from build123d import *

# Parameters (mm, degrees)
BOARD_START    = 10
BOARD_DEPTH    = 1.6
TERMINAL_START = 11.6
SKETCH2_W      = 10
SKETCH2_H      = 7.5
TERMINAL_DEPTH = 10


with BuildPart() as part:
    # Sketch1 → Board (new body)
    with BuildSketch(Plane(origin=(0, 0, 0), x_dir=(1, 0, 0), z_dir=(0, 1, 0)).offset(BOARD_START)):
        with BuildLine():
            Line((-56, -21), (-38, -21))
            ThreePointArc((-38, -21), (-37.292893219, -21.292893219), (-37, -22))
            Line((-37, -22), (-37, -38))
            ThreePointArc((-37, -38), (-37.292893219, -38.707106781), (-38, -39))
            Line((-38, -39), (-56, -39))
            ThreePointArc((-56, -39), (-56.707106781, -38.707106781), (-57, -38))
            Line((-57, -38), (-57, -22))
            ThreePointArc((-57, -22), (-56.707106781, -21.292893219), (-56, -21))
        make_face()
    extrude(amount=BOARD_DEPTH)

    # Sketch2 → Terminal (add)
    with BuildSketch(Plane(origin=(0, 0, 0), x_dir=(1, 0, 0), z_dir=(0, 1, 0)).offset(TERMINAL_START)):
        with Locations((-47, -34)):
            Rectangle(SKETCH2_W, SKETCH2_H)
    extrude(amount=TERMINAL_DEPTH)


solid = part.part
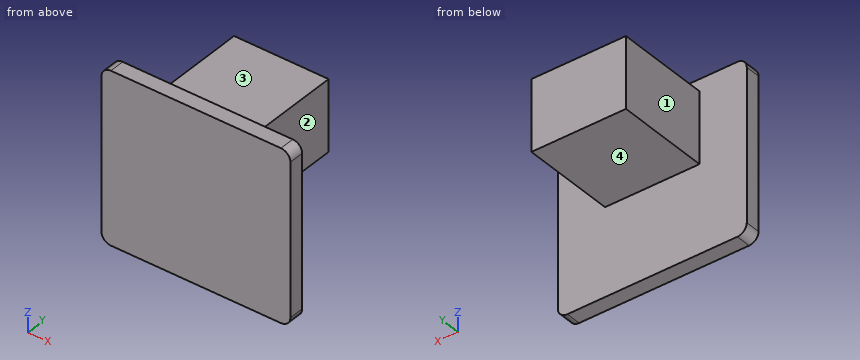
Geometry: final body of the model. Coordinates: model frame, mm. Face numbers are marked on the shaded views. A direction names the side the tool comes from. Round coordinates to 2 decimals unless told otherwise and drop trailing zeros. Order: outer loops, then holes, each group sorted by start corner. A loop starts at its lowest first (then second) coordinate and runs counter-clockwise, first axis right, second up. Notation, with made-up numbers: (2.25, 57) -> (55.25, 57) arc R11 cw to (55.25, 75) -> close; hole circle Ø8 at (88.5, 37.5). An arc over 180 degrees is marked (long way). Put each result on its own line as item: value. Start each with the question number.
Q1. Section B-B on x = -51.75. Return the cut outline in (y, z).
Q2. Section A-A on z = 33.25. Return the cut outline in (x, y), and give its area (3 significant figures).
Q3. Section C-C on y = 16.75. Return the cut outline in (x, z).
Q4. Reachability of the marked faces 1, 2, 3 and 4 from +Z, -Z, +X, -X, +Y, -Y: full face, straight path, thin tool, end or side. Return the list, or none.
Q5. Section D-D on z = 28.5. Return the cut outline in (x, y).
Q6. Line query: probe 1 along Z at (x, y) = (-48.25, 15.75); probe 2 along Y at (x, z) = (-49, 29); probe 3 along X at (y, z) = (12.25, 32). Output: solid intervals per line, ascending.
Q7. First-contact query: pin 1 (2 mm diameter, centred on y = 18, z = 32.5, fed in from +X); pin 2 (3 mm diameter, centred on x = -49, y = 17, fed in from +Z). Flat tips, straight axial feed; report the tip coordinate or a pass-through.
Ans:
1. outline: (10, 21) -> (11.6, 21) -> (11.6, 30.25) -> (21.6, 30.25) -> (21.6, 37.75) -> (11.6, 37.75) -> (11.6, 39) -> (10, 39) -> close
2. outline: (-57, 10) -> (-37, 10) -> (-37, 11.6) -> (-42, 11.6) -> (-42, 21.6) -> (-52, 21.6) -> (-52, 11.6) -> (-57, 11.6) -> close
2. area: 132 mm2
3. outline: (-52, 30.25) -> (-42, 30.25) -> (-42, 37.75) -> (-52, 37.75) -> close
4. face 1: +Z, -Z, -X, +Y
4. face 2: +Z, -Z, +X, +Y
4. face 3: +Z, +X, -X, +Y
4. face 4: -Z, +X, -X, +Y
5. outline: (-57, 10) -> (-37, 10) -> (-37, 11.6) -> (-57, 11.6) -> close
6. probe 1: z = 30.25 to 37.75
6. probe 2: y = 10 to 11.6
6. probe 3: x = -52 to -42
7. pin 1: stops at x = -42
7. pin 2: stops at z = 37.75
